```python
from build123d import *

# Parameters (mm, degrees)
SKETCH096_R         = 22
SKETCH096_R_2       = 3.1
PAD057_DEPTH        = 8
HOLE005_D           = 4.3
HOLE005_CSINK_D     = 8.298
HOLE005_CSINK_ANGLE = 82
SKETCH093_R         = 4
PAD058_DEPTH        = 1
PAD059_DEPTH        = 7
SKETCH094_R         = 1.75
POCKET029_DEPTH     = 6.001


with BuildPart() as part:
    # Sketch096 → Pad057 (new body)
    with BuildSketch(Plane.XY):
        Circle(SKETCH096_R)
        Circle(SKETCH096_R_2, mode=Mode.SUBTRACT)
    extrude(amount=PAD057_DEPTH)

    # Hole005 (through all)
    with Locations(Plane.XY.offset(8)):
        with Locations((-6.914797, 6.914797), (6.914797, 6.914797), (6.914797, -6.914797), (-6.914797, -6.914797)):
            CounterSinkHole(HOLE005_D / 2, HOLE005_CSINK_D / 2, counter_sink_angle=HOLE005_CSINK_ANGLE)

    # Sketch093 → Pad058 (join)
    with BuildSketch(Plane.XY.offset(4.5)):
        Circle(SKETCH093_R)
    extrude(amount=PAD058_DEPTH)

    # Sketch095 → Pad059 (join)
    with BuildSketch(Plane.XY.offset(1)):
        with BuildLine():
            Line((-22, 0), (-22, 28.6))
            Line((-22, 28.6), (22, 28.6))
            Line((22, 28.6), (22, 0))
            Line((22, 0), (21, 0))
            ThreePointArc((21, 0), (0, 21), (-21, 0))
            Line((-21, 0), (-22, 0))
        make_face()
    extrude(amount=PAD059_DEPTH)

    # Sketch094 → Pocket029 (cut, through all)
    with BuildSketch(Plane.XY.offset(2)):
        with Locations((-12, 18.3)):
            Circle(SKETCH094_R)
        with Locations((12, 18.3)):
            Circle(SKETCH094_R)
    extrude(amount=POCKET029_DEPTH, mode=Mode.SUBTRACT)


solid = part.part
```
Read the model definition and answer for the solid it produces. Units are mm, in the model's axes. A direction names the side the tool comes from. Give positions to 0.01 mm unless a question says otherwise; leave off trailing zeros. Write each loop counter-clockwise with the first axis right and the second up, starting at its lowest first coordinate (ties: lowest second). Pieces come first, ordered by that corner, then holes. Notation, with made-up numbers: (86, 64.25) - (97, 64.25) arc R33 ccw to (97, 92.25) - close; hole circle Ø11 at (13, 35). An arc over 180 degrees is marked (long way). Write item = value, one per line. Start each with the question number.
Item 1: Find the intervals of material crossed by probe 1 along X at (y, z) = (18.3, 6.25); probe 2 along Y at (x, z) = (0, 3.5); probe 3 along X at (y, z) = (-9.5, 6.5), in increasing order. Write a range as [from, to].
Item 2: Find section C-C (x = -2). Give the vertices of the cut face in (y, z).
Item 3: Find section A-A (z = 7). Give the vertices of the cut face in (x, y).
Item 4: A tool of negligible diameter and unlimited length cuts with its end or side. For faces 4 (the cylindrical face through (1.43, -2.75, 6.73)), 5 (the flat face through (0, 0, 4.5)), 6 (the cylindrical face through (-6.635, 9.047, 2.81)), from which of +Z, -Z, +X, -X, +Y, -Y can it reach the whole face along a straight path? Write none if from no direction.
Item 5: Find section B-B (y = 18.3). Give the vertices of the cut face in (x, z), then the cut area to 3 significant figures.
Item 6: The mould has two halves that part along X. Classify faces 1 (the flat face through (-12, 18, 2)), 2 (the flat face through (0, 24, 1)), 3 (the cylindrical face through (10.15, -19.52, 3.94)): +X half, -X half, draft (parallel to the pull), parting line (faces both ways), or undercut.
Item 7: Each of these flat-tipped pins is pushed along its axis until it touches: P1, Ø2, axis at x = -15.5, z = 4.5, coming from the -Y side; P2, Ø5.5, axis at x = 6.91, y = -6.91, coming from the +Z side; P3, Ø5.5, axis at x = 0, y = 0, coming from the +Z side; P4, Ø3.5, axis at x = -6.91, y = -6.91, coming from the -Z side. Where does it stop, or does it pass through?
Item 8: Find section D-D (x = 8.5). State how many separate pieces and enclosed holes the cut face has, then the cut area to 3 significant figures.
Response:
q1.probe_1 = [-22, -13.75], [-10.25, 10.25], [13.75, 22]
q1.probe_2 = [-22, -3.1], [3.1, 28.6]
q1.probe_3 = [-19.84, -8.1], [-5.73, 5.73], [8.1, 19.84]
q2.outline = (-21.91, 0) - (-2.37, 0) - (-2.37, 4.5) - (2.37, 4.5) - (2.37, 0) - (21.91, 0) - (21.91, 1) - (28.6, 1) - (28.6, 8) - (2.37, 8) - (2.37, 5.5) - (-2.37, 5.5) - (-2.37, 8) - (-21.91, 8) - close
q3.outline = (-22, 0) arc R22 ccw to (22, 0) - (22, 28.6) - (-22, 28.6) - close; hole circle Ø3.5 at (-12, 18.3); hole circle Ø6.56 at (-6.91, -6.91); hole circle Ø6.56 at (-6.91, 6.91); hole circle Ø6.2 at (0, 0); hole circle Ø6.56 at (6.91, -6.91); hole circle Ø6.56 at (6.91, 6.91); hole circle Ø3.5 at (12, 18.3)
q4.face_4 = +Z
q4.face_5 = -Z
q4.face_6 = +Z, -Z
q5.outline = (-22, 1) - (-12.21, 1) - (-12.21, 0) - (12.21, 0) - (12.21, 1) - (22, 1) - (22, 8) - (13.75, 8) - (13.75, 2) - (10.25, 2) - (10.25, 8) - (-10.25, 8) - (-10.25, 2) - (-13.75, 2) - (-13.75, 8) - (-22, 8) - close
q5.area = 290 mm²
q6.face_1 = undercut
q6.face_2 = draft
q6.face_3 = parting line
q7.P1 = -16.55
q7.P2 = 6.4
q7.P3 = 5.5
q7.P4 = through
q8.separate_pieces = 3
q8.enclosed_holes = 0
q8.area = 325 mm²
